Source: CAD feature listing. Evaluate the final solid. Frame: model axes, mm. A direction names the side the tool comes from. Round coordinates to 2 decimals unless told otherwise and drop trailing zeros. Loops run counter-clockwise (first coordinate to the right, second up) from the corner with the lowest first, then second, coordinate; pieces in that order, holes last.
(1) Section C-C, the plane x = -693.5. Return the cut outline in (y, z), plus the area to 3 significant figures.
(2) Section A-A, the plane y = 0. Return the cut outline in (x, z).
(3) Section B-B, the plane z = -213. Return the cut outline in (x, y).
(4) Set-up query: faces 1 (the flat face through (0, -1, 374)), 2 (the cylindrical face through (-2384.86, 34.14, -153.55)), 3 (the cylindrical face through (-1036.485, -8.266, 312.225)). Return all of +Z, -Z, +X, -X, +Y, -Y with unobstructed straight access to the full face (end or side cutting, diameter ignored); none if empty.
(5) First-contact query: pin 1 Ø1.5 at (x, y) = (-593.5, 35) entering from -Z; pin 2 Ø1.5 at (x, y) = (-1144, -2) entering from -Z; pin 3 Ø4 at (y, z) = (-3, -196.5) entering from +X. Flat tips, straight axial feed; report the tip coordinate or a pass-through.
(6) Material intervals for probe 1 along Y at (x, z) = (-2211.5, 328); probe 2 along X at (y, z) = (8, -156.5); probe 3 along Z at (x, y) = (-1143, 23), sorted ascending.
```python
from build123d import *

# Parameters (mm, degrees)
F1_R     = 63.5
F3_SIZE2 = 12.7
F3_SIZE  = 12.7


with BuildPart() as f2:
    # F2: sweep along a path in F0
    with BuildLine(Plane.XZ) as f2_path:
        Line((0, 375.1847569466), (-2032, 375.1847569466))
        ThreePointArc((-2032, 375.1847569466), (-2319.3681958742, 256.1529528208), (-2438.4, -31.2152430534))
        Line((-2438.4, -31.2152430534), (-2438.4, -285.2152430534))
    # F1 (on Right) → F2 (sweep)
    with BuildSketch(Plane.YZ):
        with Locations((0, 375.1847569466)):
            Circle(F1_R)
    sweep(path=f2_path.line)

    # F3
    f3_edges = [f2.edges().sort_by_distance(p)[0] for p in [
        (0, -63.5, 375.184757),
        (-2438.4, -63.5, -285.215243),
    ]]
    chamfer(f3_edges, length=F3_SIZE, length2=F3_SIZE2)


solid = f2.part
```
Output values:
1. outline: circle Ø127 at (0, 375.18)
1. area: 12,700 mm2
2. outline: (-2501.9, -272.52) - (-2489.2, -285.22) - (-2387.6, -285.22) - (-2374.9, -272.52) - (-2374.9, -31.22) arc R342.9 cw to (-2032, 311.68) - (-12.7, 311.68) - (0, 324.38) - (0, 425.98) - (-12.7, 438.68) - (-2032, 438.68) arc R469.9 ccw to (-2501.9, -31.22) - close
3. outline: circle Ø127 at (-2438.4, 0)
4. face 1: +Z, -Z, +X, +Y, -Y
4. face 2: -Z
4. face 3: +X
5. pin 1: stops at z = 321.71
5. pin 2: stops at z = 311.7
5. pin 3: stops at x = -2374.91
6. probe 1: y = -63.32 to 63.32
6. probe 2: x = -2501.39 to -2375.41
6. probe 3: z = 316 to 434.37
